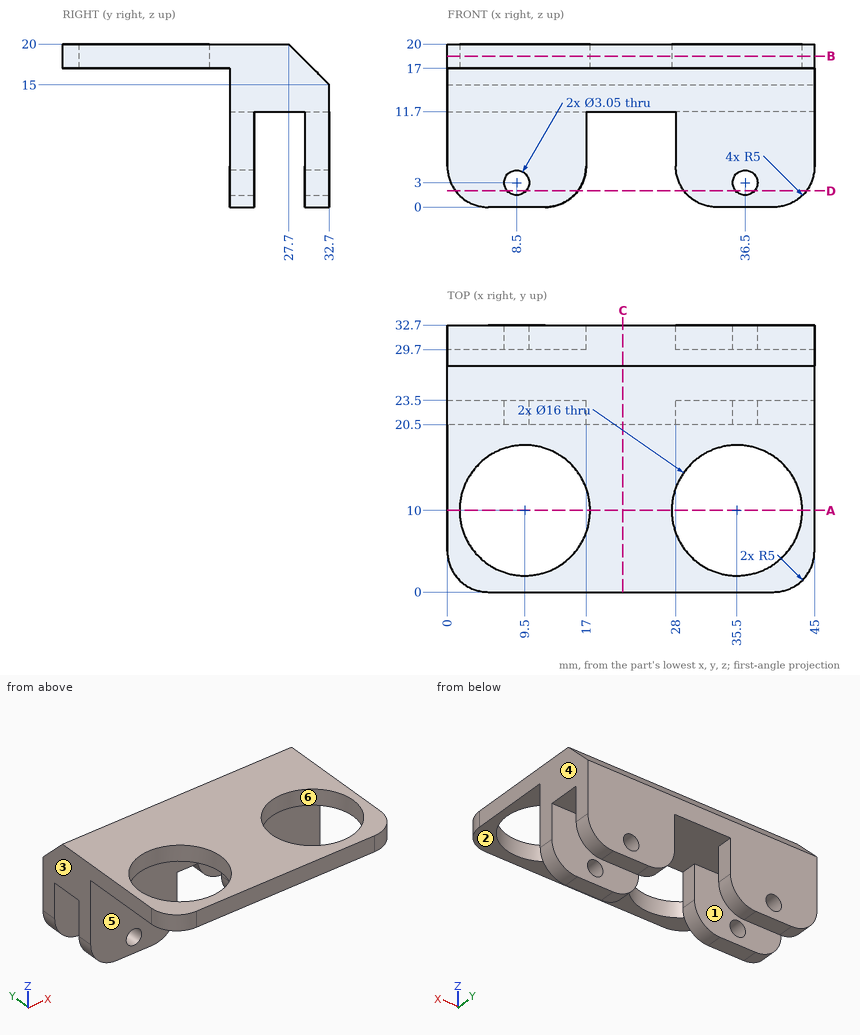
Job drawing, mm, ordinate dimensions from the low corner. One solid piece. A direction names the side the tool comes from. Round coordinates to 2 decimals unless told otherwise and drop trailing zeros. Write each loop counter-clockwise with the first axis right and the second up, starting at its lowest first coordinate (ties: lowest second). Pieces come first, ordered by that corner, then holes. Notation, with made-up numbers: (33, 31) -> (91, 31) arc R24 cw to (91, 56) -> close; hole circle Ø9 at (16, 12.5). An arc over 180 degrees is marked (long way). Answer as a JSON object with one key per item and string values.
(1) Band-saw the part on A-A, the plane y = 10. List the corners of the cut face in (x, z), then the cut area to 3 significant figures.
Reported:
{"outline": "(0, 17) -> (1.5, 17) -> (1.5, 20) -> (0, 20) -> close; (17.5, 17) -> (27.5, 17) -> (27.5, 20) -> (17.5, 20) -> close; (43.5, 17) -> (45, 17) -> (45, 20) -> (43.5, 20) -> close", "area": "39.0 mm^2"}
(2) Band-saw the part on B-B, the plane z = 18.5. List the corners of the cut face in (x, y), then the cut area to 3 significant figures.
Reported:
{"outline": "(0, 5) arc R5 ccw to (5, 0) -> (40, 0) arc R5 ccw to (45, 5) -> (45, 29.2) -> (0, 29.2) -> close; hole circle Ø16 at (9.5, 10); hole circle Ø16 at (35.5, 10)", "area": "901 mm^2"}
(3) Which spindle directions (+Z, -Z, +X, -X, +Y, -Y) get a long thin tool onto all of the face, cutting with end or side? Do the marked faces 1, 2 and 3. Say none if no direction does.
Reported:
{"face 1": "-Z, +X, -X", "face 2": "-Z, +X, -X, -Y", "face 3": "+Z, -Z, -X, +Y, -Y"}
(4) Band-saw the part on C-C, the plane x = 21.5. List the corners of the cut face in (y, z), then the cut area to 3 significant figures.
Reported:
{"outline": "(0, 17) -> (20.5, 17) -> (20.5, 11.7) -> (32.7, 11.7) -> (32.7, 15) -> (27.7, 20) -> (0, 20) -> close", "area": "150 mm^2"}
(5) Two-plate mould, pull along Y, no slides. Class the marked faces 4, 5 and 6: +Y half, -Y half, draft (parallel to the pull), parting line (faces both ways), or undercut.
Reported:
{"face 4": "draft", "face 5": "-Y half", "face 6": "undercut"}
(6) Probe probe 1 along Y at (x, z) = (36, 10); probe 2 along Z at (x, y) = (31.5, 2); probe 3 along Y at (x, z) = (26.5, 13.75). List the from-to ranges inside material, lowest first. Write a range as [from, to].
Reported:
{"probe 1": "y = [20.5, 23.5], [29.7, 32.7]", "probe 2": "z = [17, 20]", "probe 3": "y = [20.5, 32.7]"}
(7) Band-saw the part on D-D, the plane z = 2. Count the separate pieces of the cut face and the enclosed holes in it, then the cut area to 3 significant figures.
Reported:
{"separate pieces": "8", "enclosed holes": "0", "area": "152 mm^2"}
(8) Pin check, flat tips, straight feed: P1, Ø16.5, axis at x = 13.5, y = 6.5, coming from the -Z side; P2, Ø6, axis at x = 6, z = 8, coming from the -Y side; P3, Ø6, axis at x = 17, y = 28, coming from the -Z side. Stop position of each tip, or through.
Reported:
{"P1": "stops at z = 17", "P2": "stops at y = 20.5", "P3": "stops at z = 0.69"}
